Input: part model. Units: mm. Frame: model coordinates. Face numbers are marked on the shaded views. A direction names the side the tool comes from. Coordinates: 2 decimals unless noted, no trailing zeros. Loops run counter-clockwise (first coordinate to the right, second up) from the corner with the lowest first, then second, coordinate; pieces in that order, holes last. Notation, with made-up numbers: M 50,85.5 L 69,85.5 A21 ccw 69,121.5 Z; hole C -11,76.5 d3. An arc over 180 degrees is marked long. Use a Markdown table: item, result. Add a question column.
1. Line query: L1, parallel to X at y = 0.4, z = -20; L2, parallel to X at y = -0.45, z = -66; L3, parallel to X at y = 0.5, z = -36.5. Output: solid intervals per line, ascending. Write a range as [from, to].
2. Pin query (flat end, axial travel): pin 1 (2 mm diameter, centred on y = 1.5, z = -17.5, fed in from -X); pin 2 (3 mm diameter, centred on x = -1, y = 0.5, fed in from -Z); pin 3 (0.5 mm diameter, centred on y = 0.5, z = -42.5, fed in from -X). Return the tip coordinate at first contact, or that it passes through.
3. Set-up query: the marked faces 1 and 2. Return all of +Z, -Z, +X, -X, +Y, -Y with unobstructed straight access to the full face (end or side cutting, diameter ignored); none if empty.
4. Section B-B on z = -45. Output: boundary loops of the cut face in (x, y).
5. Section A-A on x = 0. Output: boundary loops of the cut face in (y, z).
6. Section C-C on x = 43. Output: boundary loops of the cut face in (y, z), then the cut area to 3 significant figures.
```python
from build123d import *

# Parameters (mm, degrees)
SKETCH3_R           = 3
SKETCH3_R_2         = 2
SKETCH3_W           = 211
SKETCH3_H           = 1
BOSS_EXTRUDE2_DEPTH = 80
SKETCH3_18_R        = 3
CUT_EXTRUDE1_DEPTH  = 5
BOSS_EXTRUDE3_START = -5
SKETCH3_19_R        = 2
BOSS_EXTRUDE3_DEPTH = 75
CUT_EXTRUDE2_START  = -5
SKETCH3_20_R        = 3
SKETCH3_20_R_2      = 2
CUT_EXTRUDE2_DEPTH  = 5
CUT_EXTRUDE3_START  = -17.5
SKETCH3_21_R        = 3
SKETCH3_21_R_2      = 2
CUT_EXTRUDE3_DEPTH  = 5
CUT_EXTRUDE4_START  = -22.5
SKETCH3_22_R        = 3
CUT_EXTRUDE4_DEPTH  = 35
CUT_EXTRUDE5_START  = -57.5
SKETCH3_23_R        = 3
SKETCH3_23_R_2      = 2
CUT_EXTRUDE5_DEPTH  = 5
CUT_EXTRUDE8_START  = -70
SKETCH3_26_R        = 3
SKETCH3_26_R_2      = 2
CUT_EXTRUDE8_DEPTH  = 5
CUT_EXTRUDE9_START  = -75
SKETCH3_27_R        = 3
CUT_EXTRUDE9_DEPTH  = 5
SKETCH4_W           = 185.171572875
SKETCH4_H           = 55
CUT_EXTRUDE10_DEPTH = 228.563178041
CUT_EXTRUDE11_START = -57.5
SKETCH3_28_R        = 2
CUT_EXTRUDE11_DEPTH = 5
FILLET4_R           = 5


with BuildPart() as part:
    # Sketch3 → Boss-Extrude2 (new body)
    # profile 1 of 2: a face of its own
    with BuildSketch(Plane.XY):
        Circle(SKETCH3_R)
        Circle(SKETCH3_R_2, mode=Mode.SUBTRACT)
    # profile 2 of 2: a face of its own
    with BuildSketch(Plane.XY):
        with Locations((107.5, 0.5)):
            Rectangle(SKETCH3_W, SKETCH3_H)
    extrude(amount=-BOSS_EXTRUDE2_DEPTH)

    # Sketch3_18 → Cut-Extrude1 (cut)
    with BuildSketch(Plane.XY):
        Circle(SKETCH3_18_R)
    extrude(amount=-CUT_EXTRUDE1_DEPTH, mode=Mode.SUBTRACT)

    # Sketch3_19 → Boss-Extrude3 (add)
    with BuildSketch(Plane.XY.offset(BOSS_EXTRUDE3_START)):
        Circle(SKETCH3_19_R)
    extrude(amount=-BOSS_EXTRUDE3_DEPTH)

    # Sketch3_20 → Cut-Extrude2 (cut)
    with BuildSketch(Plane.XY.offset(CUT_EXTRUDE2_START)):
        Circle(SKETCH3_20_R)
        Circle(SKETCH3_20_R_2, mode=Mode.SUBTRACT)
    extrude(amount=-CUT_EXTRUDE2_DEPTH, mode=Mode.SUBTRACT)

    # Sketch3_21 → Cut-Extrude3 (cut)
    with BuildSketch(Plane.XY.offset(CUT_EXTRUDE3_START)):
        Circle(SKETCH3_21_R)
        Circle(SKETCH3_21_R_2, mode=Mode.SUBTRACT)
    extrude(amount=-CUT_EXTRUDE3_DEPTH, mode=Mode.SUBTRACT)

    # Sketch3_22 → Cut-Extrude4 (cut)
    with BuildSketch(Plane.XY.offset(CUT_EXTRUDE4_START)):
        Circle(SKETCH3_22_R)
    extrude(amount=-CUT_EXTRUDE4_DEPTH, mode=Mode.SUBTRACT)

    # Sketch3_23 → Cut-Extrude5 (cut)
    with BuildSketch(Plane.XY.offset(CUT_EXTRUDE5_START)):
        Circle(SKETCH3_23_R)
        Circle(SKETCH3_23_R_2, mode=Mode.SUBTRACT)
    extrude(amount=-CUT_EXTRUDE5_DEPTH, mode=Mode.SUBTRACT)

    # Sketch3_26 → Cut-Extrude8 (cut)
    with BuildSketch(Plane.XY.offset(CUT_EXTRUDE8_START)):
        Circle(SKETCH3_26_R)
        Circle(SKETCH3_26_R_2, mode=Mode.SUBTRACT)
    extrude(amount=-CUT_EXTRUDE8_DEPTH, mode=Mode.SUBTRACT)

    # Sketch3_27 → Cut-Extrude9 (cut)
    with BuildSketch(Plane.XY.offset(CUT_EXTRUDE9_START)):
        Circle(SKETCH3_27_R)
    extrude(amount=-CUT_EXTRUDE9_DEPTH, mode=Mode.SUBTRACT)

    # Sketch4 → Cut-Extrude10 (cut, through all)
    with BuildSketch(Plane(origin=(0, 1, 0), x_dir=(1, 0, 0), z_dir=(0, 1, 0))):
        with Locations((107.914213562, 40)):
            Rectangle(SKETCH4_W, SKETCH4_H)
    extrude(amount=-CUT_EXTRUDE10_DEPTH, mode=Mode.SUBTRACT)

    # Sketch3_28 → Cut-Extrude11 (cut)
    with BuildSketch(Plane.XY.offset(CUT_EXTRUDE11_START)):
        Circle(SKETCH3_28_R)
    extrude(amount=-CUT_EXTRUDE11_DEPTH, mode=Mode.SUBTRACT)

    # Fillet4
    fillet4_edges = [part.edges().sort_by_distance(p)[0] for p in [
        (200.5, 0.5, -12.5),
        (15.328427125, 0.5, -12.5),
        (15.328427125, 0.5, -67.5),
        (200.5, 0.5, -67.5),
    ]]
    fillet(fillet4_edges, radius=FILLET4_R)


solid = part.part
```
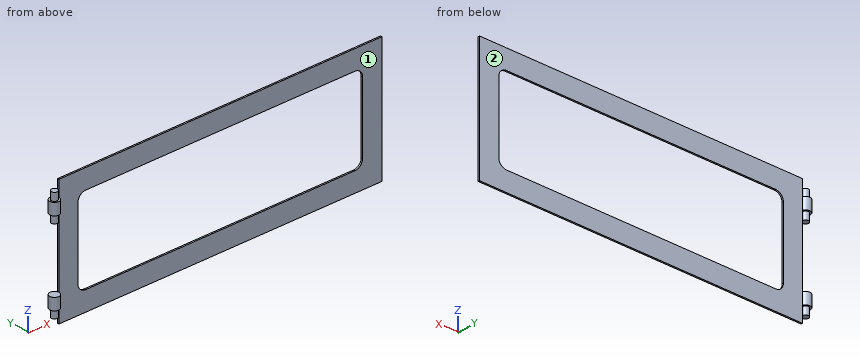
Answers below:
| question | item | result |
|---|---|---|
| 1 | L1 | x = [-1.96, 1.96], [2.97, 15.33], [200.5, 213] |
| 1 | L2 | x = [-2.97, 2.97] |
| 1 | L3 | x = [2.96, 15.33], [200.5, 213] |
| 2 | pin 1 | stops at x = -2.96 |
| 2 | pin 2 | stops at z = -75 |
| 2 | pin 3 | stops at x = 2.9 |
| 3 | face 1 | +Z, -Z, +X, -Y |
| 3 | face 2 | +Z, -Z, +X, +Y |
| 4 | outline | M 2.83,1 A3 cw 3,0 L 15.33,0 L 15.33,1 Z; M 200.5,0 L 213,0 L 213,1 L 200.5,1 Z |
| 5 | outline | M -3,-70 L -2,-70 L -2,-75 L 2,-75 L 2,-70 L 3,-70 L 3,-62.5 L -3,-62.5 Z; M -3,-17.5 L -2,-17.5 L -2,-22.5 L 2,-22.5 L 2,-17.5 L 3,-17.5 L 3,-10 L 2,-10 L 2,-5 L -2,-5 L -2,-10 L -3,-10 Z |
| 6 | outline | M 0,-80 L 1,-80 L 1,-67.5 L 0,-67.5 Z; M 0,-12.5 L 1,-12.5 L 1,0 L 0,0 Z |
| 6 | area | 25.0 mm² |
